```python
from build123d import *

# Parameters (mm, degrees)
F4_R     = 3.175
F5_DEPTH = 12.7


# Not quite as in the source:
# - a fillet or chamfer that OpenCascade refuses, or shapes differently, is made with other operations: its cross-section is extruded or revolved along the edge and cut away or added


with BuildPart() as f1:
    # F0 (on Front) → F1 (revolve)
    with BuildSketch(Plane.XZ):
        Polygon((0, 7.9375), (5.6608929044, 7.8860616331), (29.5304771808, 25.4019652116), (29.337, 34.925), (15.3162, 34.925), (15.3162, 32.385), (12.7, 32.385), (12.7, 34.925), (0, 34.925), align=None)
    revolve(axis=Axis((10.2213714272, 0, 0), (1, 0, 0)))

    # F2: chamfer of 1.905 on 2 edges, made by hand

    # F2_s1 → F2_t2 (revolve, cut)
    with BuildSketch(Plane.XZ):
        Polygon((1.905, 34.925), (0, 33.02), (0, 34.925), align=None)
    revolve(axis=Axis((0, 0, 0), (1, 0, 0)), mode=Mode.SUBTRACT)

    # F2_s3 → F2_t4 (revolve, cut)
    with BuildSketch(Plane.XZ):
        Polygon((29.3749172557, 33.0586954362), (27.4703102981, 34.925), (29.337, 34.925), align=None)
    revolve(axis=Axis((29.337, 0, 0), (1, 0, 0)), mode=Mode.SUBTRACT)

    # F4 (on offset) → F5 (cut)
    with BuildSketch(Plane.YZ.offset(33.655)):
        with Locations((20.9239967621, 20.9239967621)):
            Circle(F4_R)
        with Locations((20.9239967621, -20.9239967621)):
            Circle(F4_R)
        with Locations((-20.9239967621, -20.9239967621)):
            Circle(F4_R)
        with Locations((-20.9239967621, 20.9239967621)):
            Circle(F4_R)
    extrude(amount=-F5_DEPTH, mode=Mode.SUBTRACT)


solid = f1.part
```
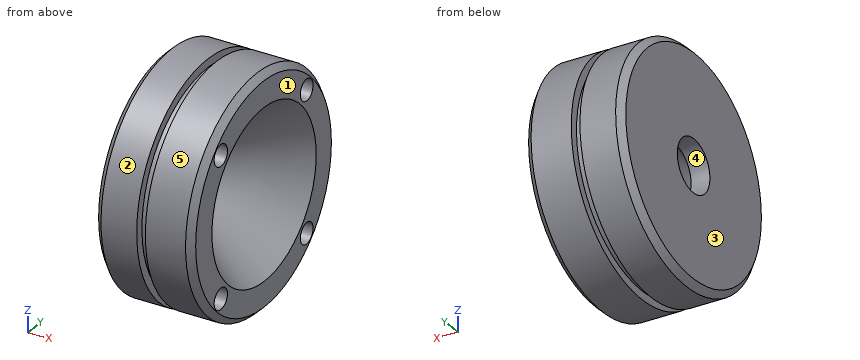
Verification items for the finished model (mm, model axes). Face numbers are marked on the shaded views. A direction names the side the tool comes from. Give positions to 0.01 mm unless a question says otherwise; leave off trailing zeros. Loops run counter-clockwise (first coordinate to the right, second up) from the corner with the lowest first, then second, coordinate; pieces in that order, holes last. Notation, with made-up numbers: M 64,44.25 L 107,44.25 A9 cw 107,48.25 Z; hole C 60,46 d4. An arc over 180 degrees is marked long. Return JSON: item names as keys, results as strings.
1) Tool access check on the marked faces 1 and 2. Record the directions out of +Z, -Z, +X, -X, +Y, -Y that give a thin tool (end or side, any length) a straight path to the whole face; none if there is none.
Findings:
{"face 1": "+X", "face 2": "+X, -X"}
2) Section check C-C, the plane x = 4. Enter the section's corners in (y, z) (3 decimals).
Findings:
{"outline": "C 0,0 d69.85; hole C 0,0 d15.802"}
3) Section check A-A, the plane x = 24.5. Enter the section's corners in (y, z) (3 decimals), and give its area (3 significant figures).
Findings:
{"outline": "C 0,0 d69.85; hole C -20.924,-20.924 d6.35; hole C -20.924,20.924 d6.35; hole C 0,0 d43.421; hole C 20.924,-20.924 d6.35; hole C 20.924,20.924 d6.35", "area": "2,220 mm2"}
4) Section check B-B, the plane x = 16.25. Enter the section's corners in (y, z) (3 decimals), and give its area (3 significant figures).
Findings:
{"outline": "C 0,0 d69.85; hole C 0,0 d31.313", "area": "3,060 mm2"}
5) Mould release check, pull along Z, two halves, no side actions. Record for the marked faces 3, 4 and 5: released by +Z, released by -Z, zero draft, split by the parting line, or undercut.
Findings:
{"face 3": "zero draft", "face 4": "undercut", "face 5": "split by the parting line"}
6) Gauge pin test, flat ends, axial feed: P1, Ø12, axis at x = 13.5, z = -3, coming from the +Y side (3 decimals); P2, Ø10, axis at x = 25, y = -7.5, coming from the +Z side; P3, Ø3, axis at y = 19.5, z = 22, coming from the +X side. Record the tip position at first contact, or that the pin passes through.
Findings:
{"P1": "stops at y = 34.925", "P2": "stops at z = 34.84", "P3": "stops at x = 29.47"}
7) Material ranges on L1, parallel to X at y = -22, z = 24; L2, parallel to Z at x = 12.25, y = -9.5; L3, parallel to Z at x = 12.25, y = -7.5, recorded low to high. Write a range as [from, to].
Findings:
{"L1": "x = [0, 12.7], [15.32, 29.39]", "L2": "z = [-33.61, -8.46], [8.46, 33.61]", "L3": "z = [-34.11, -10.28], [10.28, 34.11]"}
